Work out the finished part from the listing and answer in its coordinate system (mm). Face numbers are marked on the shaded views. A direction names the side the tool comes from. Coordinates: 2 decimals unless noted, no trailing zeros. Order: outer loops, then holes, each group sorted by start corner. A loop starts at its lowest first (then second) coordinate and runs counter-clockwise, first axis right, second up.
1. Determine the mould class of the marked faces 6, 7 and 8 for opening direction Z: +Z half, -Z half, draft (parallel to the pull), parting line (faces both ways), or undercut.
2. The part is cut by section B-B, the plane y = -25. Give the vertices of the cut face in (x, z), then the cut area to 3 significant figures.
3. Flat-ended cylindrical pins translate along their axes: pin 1 Ø2.5 at (y, z) = (25, 2) entering from -X; pin 2 Ø3 at (y, z) = (-10, 10) entering from -X; pin 3 Ø6 at (x, z) = (-10.5, 14.5) entering from -Y; pin 4 Ø6.5 at (y, z) = (-10, -10) entering from +X. Find the tip coordinate at first contact, or state that the pin passes through.
4. Find the intervals of material crossed by probe 1 along Z at (x, y) = (-28, -10); probe 2 along Y at (x, z) = (5.5, -7.5); probe 3 along Z at (x, y) = (-31, -10), in increasing order.
5. The part is cut by section D-D, the plane y = 11. Give the vertices of the cut face in (x, z), then the cut area to 3 significant figures.
6. The part is cut by section C-C, the plane z = -3. Give the vertices of the cut face in (x, y).
7. The part is cut by section A-A, the plane x = 14. Give the vertices of the cut face in (y, z), then the cut area to 3 significant figures.
8. A tool of negligible diameter and unlimited length cuts with its end or side. For the marked faces 1, 2, 3, 4 and 5, from which of +Z, -Z, +X, -X, +Y, -Y can it reach the whole face along a straight path? Write none if from no direction.
```python
from build123d import *

# Parameters (mm, degrees)
SKETCH1_W           = 45
SKETCH1_H           = 40
BOSS_EXTRUDE1_DEPTH = 28
SKETCH5_W           = 30
SKETCH5_H           = 18
CUT_EXTRUDE2_DEPTH  = 40
SKETCH6_W           = 8.5
SKETCH6_H           = 5
CUT_EXTRUDE3_DEPTH  = 17
SKETCH7_W           = 9
SKETCH7_H           = 6
CUT_EXTRUDE4_DEPTH  = 17
SKETCH8_W           = 45
SKETCH8_H           = 40
BOSS_EXTRUDE2_DEPTH = 5
SKETCH9_W           = 40
SKETCH9_H           = 10
BOSS_EXTRUDE3_DEPTH = 10
SKETCH10_W          = 5
SKETCH10_H          = 40
BOSS_EXTRUDE4_DEPTH = 30
SKETCH13_R          = 2.5
CUT_EXTRUDE5_DEPTH  = 27
FILLET1_R           = 10
FILLET3_R           = 7
FILLET4_R           = 7


with BuildPart() as part:
    # Sketch1 → Boss-Extrude1 (new body)
    with BuildSketch(Plane(origin=(0, 0, 0), x_dir=(1, 0, 0), z_dir=(0, 1, 0))):
        Rectangle(SKETCH1_W, SKETCH1_H)
    extrude(amount=BOSS_EXTRUDE1_DEPTH)

    # Sketch5 → Cut-Extrude2 (cut)
    with BuildSketch(Plane.ZY.offset(22.5)):
        with Locations((0, 14)):
            Rectangle(SKETCH5_W, SKETCH5_H)
    extrude(amount=-CUT_EXTRUDE2_DEPTH, mode=Mode.SUBTRACT)

    # Sketch6 → Cut-Extrude3 (cut)
    with BuildSketch(Plane.ZY.offset(22.5)):
        with Locations((0, 25.5)):
            Rectangle(SKETCH6_W, SKETCH6_H)
    extrude(amount=-CUT_EXTRUDE3_DEPTH, mode=Mode.SUBTRACT)

    # Sketch7 → Cut-Extrude4 (cut)
    with BuildSketch(Plane(origin=(22.5, 0, 0), x_dir=(0, 0, -1), z_dir=(1, 0, 0))):
        with Locations((0, 9)):
            Rectangle(SKETCH7_W, SKETCH7_H)
    extrude(amount=-CUT_EXTRUDE4_DEPTH, mode=Mode.SUBTRACT)

    # Sketch8 → Boss-Extrude2 (add)
    with BuildSketch(Plane.XZ):
        Rectangle(SKETCH8_W, SKETCH8_H)
    extrude(amount=BOSS_EXTRUDE2_DEPTH)

    # Sketch9 → Boss-Extrude3 (add)
    with BuildSketch(Plane.ZY.offset(22.5)):
        Rectangle(SKETCH9_W, SKETCH9_H)
    extrude(amount=BOSS_EXTRUDE3_DEPTH)

    # Sketch10 → Boss-Extrude4 (add)
    with BuildSketch(Plane.XZ.offset(5)):
        with Locations((-30, 0)):
            Rectangle(SKETCH10_W, SKETCH10_H)
    extrude(amount=BOSS_EXTRUDE4_DEPTH)

    # Sketch13 → Cut-Extrude5 (cut)
    with BuildSketch(Plane.ZY.offset(32.5)):
        with Locations((-10, -25)):
            Circle(SKETCH13_R)
        with Locations((-10, -10)):
            Circle(SKETCH13_R)
        with Locations((10, -10)):
            Circle(SKETCH13_R)
        with Locations((10, -25)):
            Circle(SKETCH13_R)
    extrude(amount=-CUT_EXTRUDE5_DEPTH, mode=Mode.SUBTRACT)

    # Fillet1
    # the kernel refuses this fillet: 10 mm, written as the material it adds along each edge
    with BuildSketch(Plane(origin=(-27.5, -5, 20), x_dir=(0, -1, 0), z_dir=(0, 0, -1))) as fillet1_piece_1_section:
        with BuildLine():
            CenterArc((FILLET1_R, -FILLET1_R), FILLET1_R, 90, 90)
            Line((0, -FILLET1_R), (0, 0))
            Line((0, 0), (FILLET1_R, 0))
        make_face()
    fillet1_piece_1 = extrude(amount=40, mode=Mode.PRIVATE)
    fillet1_piece_1 = fillet1_piece_1 - Plane(origin=(-25.136048253, -10, 10), x_dir=(0, 0, 1), z_dir=(-1, 0, 0)) * Cylinder(2.5, 121, mode=Mode.PRIVATE)
    fillet1_piece_1 = fillet1_piece_1 - Plane(origin=(-25.136048253, -10, -10), x_dir=(0, 0, 1), z_dir=(-1, 0, 0)) * Cylinder(2.5, 121, mode=Mode.PRIVATE)
    add(fillet1_piece_1)

    # Fillet3
    # the kernel refuses this fillet: 7 mm, written as the material it takes off along each edge
    with BuildSketch(Plane(origin=(-27.5, -15, -20), x_dir=(-1, 0, 0), z_dir=(0, -1, 0))) as fillet3_piece_1:
        with BuildLine():
            CenterArc((FILLET3_R, -FILLET3_R), FILLET3_R, 90, 90)
            Line((0, -FILLET3_R), (0, 0))
            Line((0, 0), (FILLET3_R, 0))
        make_face()
    extrude(amount=37.5, mode=Mode.SUBTRACT)
    with BuildSketch(Plane(origin=(-17.5, -15, -20), x_dir=(-1, 0, 0), z_dir=(0, -1, 0))) as fillet3_piece_2:
        with BuildLine():
            CenterArc((10 + FILLET3_R, -FILLET3_R), FILLET3_R, 90, 90)
            Line((10 + FILLET3_R, 0), (10, 0))
            Line((10, 0), (10, -FILLET3_R))
        make_face()
    revolve(axis=Axis((-17.5, -15, -20), (0, 0, -1)), revolution_arc=90, mode=Mode.SUBTRACT)
    with BuildSketch(Plane(origin=(-27.5, -15, 20), x_dir=(-1, 0, 0), z_dir=(0, -1, 0))) as fillet3_piece_3:
        with BuildLine():
            CenterArc((FILLET3_R, FILLET3_R), FILLET3_R, 180, 90)
            Line((0, FILLET3_R), (0, 0))
            Line((0, 0), (FILLET3_R, 0))
        make_face()
    extrude(amount=37.5, mode=Mode.SUBTRACT)
    with BuildSketch(Plane(origin=(-17.5, -15, 20), x_dir=(-1, 0, 0), z_dir=(0, -1, 0))) as fillet3_piece_4:
        with BuildLine():
            CenterArc((10 + FILLET3_R, FILLET3_R), FILLET3_R, 180, 90)
            Line((10 + FILLET3_R, 0), (10, 0))
            Line((10, 0), (10, FILLET3_R))
        make_face()
    revolve(axis=Axis((-17.5, -15, 20), (0, 0, -1)), revolution_arc=90, mode=Mode.SUBTRACT)
    with BuildSketch(Plane(origin=(40, -5, -20), x_dir=(0, 0, 1), z_dir=(-1, 0, 0))) as fillet3_piece_5:
        with BuildLine():
            CenterArc((FILLET3_R, FILLET3_R), FILLET3_R, 180, 90)
            Line((0, FILLET3_R), (0, 0))
            Line((0, 0), (FILLET3_R, 0))
        make_face()
    extrude(amount=57.5, mode=Mode.SUBTRACT)
    with BuildSketch(Plane(origin=(40, 28, -20), x_dir=(0, 0, 1), z_dir=(-1, 0, 0)), Plane(origin=(-40, 28, 20), x_dir=(0, 0, -1), z_dir=(1, 0, 0))) as fillet3_piece_6:
        with BuildLine():
            CenterArc((FILLET3_R, -FILLET3_R), FILLET3_R, 90, 90)
            Line((0, -FILLET3_R), (0, 0))
            Line((0, 0), (FILLET3_R, 0))
        make_face()
    extrude(amount=80, mode=Mode.SUBTRACT)
    with BuildSketch(Plane(origin=(40, -5, 20), x_dir=(0, 0, -1), z_dir=(-1, 0, 0))) as fillet3_piece_7:
        with BuildLine():
            CenterArc((FILLET3_R, -FILLET3_R), FILLET3_R, 90, 90)
            Line((0, -FILLET3_R), (0, 0))
            Line((0, 0), (FILLET3_R, 0))
        make_face()
    extrude(amount=57.5, mode=Mode.SUBTRACT)

    # Fillet4
    fillet4_edges = [part.edges().sort_by_distance(p)[0] for p in [
        (-32.5, 5, 0),
    ]]
    fillet(fillet4_edges, radius=FILLET4_R)


solid = part.part
```
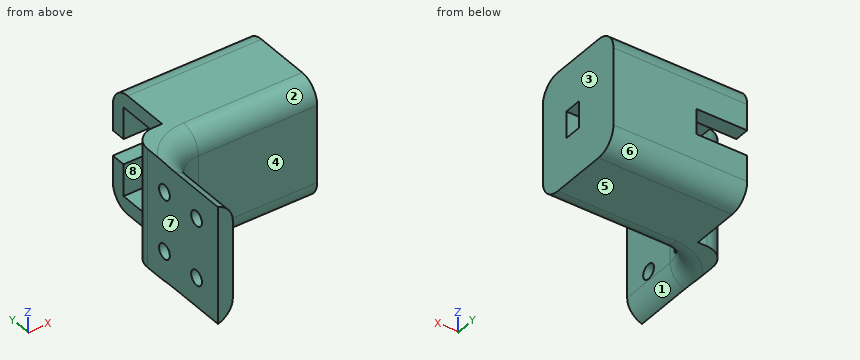
Geometry says:
1. face 6: -Z half
1. face 7: draft
1. face 8: undercut
2. outline: (-32.5, -19.71) arc R7 ccw to (-27.5, -13) - (-27.5, -12.5) - (-32.5, -12.5) - close; (-32.5, -7.5) - (-27.5, -7.5) - (-27.5, 7.5) - (-32.5, 7.5) - close; (-32.5, 12.5) - (-27.5, 12.5) - (-27.5, 13) arc R7 ccw to (-32.5, 19.71) - close
2. area: 129 mm2
3. pin 1: stops at x = -5.5
3. pin 2: passes through
3. pin 3: stops at y = -5
3. pin 4: stops at x = -23.15
4. probe 1: z = -17.49 to -12.5, -7.5 to 7.5, 12.5 to 17.49
4. probe 2: y = -5 to 5, 23 to 28
4. probe 3: z = -19.5 to -12.5, -7.5 to 7.5, 12.5 to 19.5
5. outline: (-22.5, -20) - (22.5, -20) - (22.5, -4.5) - (17.5, -4.5) - (17.5, -15) - (-22.5, -15) - close; (-22.5, 15) - (17.5, 15) - (17.5, 4.5) - (22.5, 4.5) - (22.5, 20) - (-22.5, 20) - close
5. area: 555 mm2
6. outline: (-32.5, -35) - (-27.5, -35) - (-27.5, -15) arc R10 cw to (-17.5, -5) - (22.5, -5) - (22.5, 6) - (17.5, 6) - (17.5, 5) - (-25.5, 5) arc R7 ccw to (-32.5, -2) - close; (-5.5, 23) - (17.5, 23) - (17.5, 12) - (22.5, 12) - (22.5, 28) - (-5.5, 28) - close
7. outline: (-5, -13) arc R7 ccw to (2, -20) - (21, -20) arc R7 ccw to (28, -13) - (28, 13) arc R7 ccw to (21, 20) - (2, 20) arc R7 ccw to (-5, 13) - close; hole (5, -15) - (23, -15) - (23, 15) - (5, 15) - close
7. area: 738 mm2
8. face 1: -Z, +X, -Y
8. face 2: +Z, +X, -Y
8. face 3: +Z, -Z, +X, +Y, -Y
8. face 4: +Z, -Z, +X, -Y
8. face 5: -Z, +X, -X, +Y, -Y
